Design review of the part built by this model. Coordinates are the model's own, in mm. Face numbers are marked on the shaded views. A direction names the side the tool comes from. Round coordinates to 2 decimals unless told otherwise and drop trailing zeros. Order: outer loops, then holes, each group sorted by start corner. A loop starts at its lowest first (then second) coordinate and runs counter-clockwise, first axis right, second up. Notation, with made-up numbers: (63.5, 45) - (72.5, 45) arc R18 ccw to (72.5, 59) - close; hole circle Ø7 at (59, 70.25). An arc over 180 degrees is marked (long way). Write item = value, one per line.
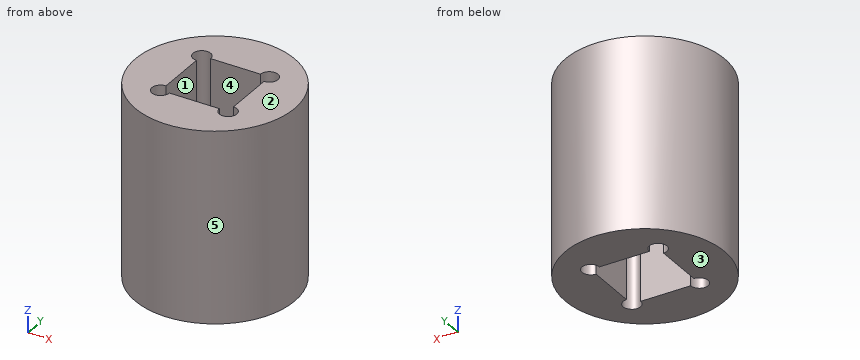
from build123d import *

# Parameters (mm, degrees)
F0_R     = 7.5
F1_DEPTH = 18


with BuildPart() as f1:
    # F0 (on Top) → F1 (new body)
    with BuildSketch(Plane.XY):
        Circle(F0_R)
        with BuildLine():
            ThreePointArc((3.175, -2.3495), (3.758717, -3.758717), (2.3495, -3.175))
            Line((2.3495, -3.175), (-2.3495, -3.175))
            ThreePointArc((-2.3495, -3.175), (-3.758717, -3.758717), (-3.175, -2.3495))
            Line((-3.175, -2.3495), (-3.175, 2.3495))
            ThreePointArc((-3.175, 2.3495), (-3.758717, 3.758717), (-2.3495, 3.175))
            Line((-2.3495, 3.175), (2.3495, 3.175))
            ThreePointArc((2.3495, 3.175), (3.758717, 3.758717), (3.175, 2.3495))
            Line((3.175, 2.3495), (3.175, -2.3495))
        make_face(mode=Mode.SUBTRACT)
    extrude(amount=F1_DEPTH)


solid = f1.part
Item 1: Insertion check: P1, Ø2, axis at x = -3.175, y = 3.175, coming from the -Z side; P2, Ø1.4, axis at x = -1, z = 9.5, coming from the -Y side; P3, Ø2, axis at x = -4, z = 13.5, coming from the +Y side; P4, Ø5, axis at x = -6, z = 5, coming from the -Y side. Each pin has a flat end and moves straight along its axis. Give the tip position at first contact, or say it passes through.
Data:
P1 = 0
P2 = -7.49
P3 = 6.87
P4 = -6.63
Item 2: Take a section at A-A, the plane x = 0. State the section outline as (y, z) points (3 decimals).
Data:
outline = (-7.5, 0) - (-3.175, 0) - (-3.175, 18) - (-7.5, 18) - close; (3.175, 0) - (7.5, 0) - (7.5, 18) - (3.175, 18) - close
Item 3: Take a section at B-B, the plane z = 1.5. State the section outline as (x, y) points (1 decimal), and give its area (3 significant figures).
Data:
outline = circle Ø15 at (0, 0); hole (-3.2, -2.3) arc R0.8 ccw (long way) to (-2.3, -3.2) - (2.3, -3.2) arc R0.8 ccw (long way) to (3.2, -2.3) - (3.2, 2.3) arc R0.8 ccw (long way) to (2.3, 3.2) - (-2.3, 3.2) arc R0.8 ccw (long way) to (-3.2, 2.3) - close
area = 130 mm2
Item 4: For the marked faces 1 and 2, list the 3-axis set-ups (+Z, -Z, +X, -X, +Y, -Y) from which the entire face can be reached by the end or side of a thin tool; tool diameter is ignored.
Data:
face_1 = +Z, -Z
face_2 = +Z, +X, -X, +Y, -Y
Item 5: The part is to be moulded in two halves that separate along X. For the marked faces 3, 4 and 5, say which applies: +X half, -X half, draft (parallel to the pull), parting line (faces both ways), or undercut.
Data:
face_3 = draft
face_4 = undercut
face_5 = parting line
Item 6: For line 1 along Y through (x, z) = (0.25, 11.75) (3 decimals); line 2 along Y through (x, z) = (1.5, 13.5) (3 decimals); line 3 along X through (y, z) = (-1, 9.5) (3 decimals), list the stretches that pass through material, from the lowest coordinate up. Write a range as [from, to].
Data:
line_1 = [-7.496, -3.175], [3.175, 7.496]
line_2 = [-7.348, -3.175], [3.175, 7.348]
line_3 = [-7.433, -3.175], [3.175, 7.433]
Item 7: Take a section at D-D, the plane x = 3.75. State the section outline as (y, z) points, and give its area (3 significant figures).
Data:
outline = (-6.5, 0) - (-3.77, 0) - (-3.77, 18) - (-6.5, 18) - close; (-2.58, 0) - (2.58, 0) - (2.58, 18) - (-2.58, 18) - close; (3.77, 0) - (6.5, 0) - (6.5, 18) - (3.77, 18) - close
area = 191 mm2
